The model under review builds one solid part; all positions refer to its coordinate system, in mm. Face numbers are marked on the shaded views. A direction names the side the tool comes from. Round coordinates to 2 decimals unless told otherwise and drop trailing zeros. Write each loop counter-clockwise with the first axis right and the second up, starting at its lowest first coordinate (ties: lowest second). Pieces come first, ordered by that corner, then holes.
Item 1: Clearance check with flat-ended pins moving along their axes: pin 1 Ø0.8 at (x, z) = (-22, -4) entering from -Y; pin 2 Ø2 at (x, y) = (-23, -11) entering from -Z; pin 3 Ø3 at (x, y) = (22.5, -14.5) entering from +Z. State where each tip first meets the part, or that it passes through.
Item 2: Draft analysis for pull direction X (two halves, no side actions). For the marked faces 1, 2 and 3, state which applies: +X half, -X half, draft (parallel to the pull), parting line (faces both ways), or undercut.
Item 3: Add section D-D (x = 31). Give the boundary of the cut face in (y, z).
Item 4: Add section A-A (y = -11.25). Give the boundary of the cut face in (x, z).
Item 5: Add section C-C (y = -21). Give the boundary of the cut face in (x, z), plus the area to 3 significant figures.
Item 6: To check wall thickness, follow L1, parallel to Z at x = -63, y = -11; L2, parallel to X at y = -34, z = 5; L3, parallel to X at y = -39.5, z = 9. State the ranges of each line that lie inside material, in increasing order.
Item 7: Add section B-B (y = -43). Give the boundary of the cut face in (x, z).
Item 8: Machinability: for the marked faces 4 and 5, which of the approach directions +Z, -Z, +X, -X, +Y, -Y give a long, thin tool a straight path to every point of the face, cutting with its end or side? Answer none if there is none.
```python
from build123d import *
from build123d import SkipClean  # not in build123d's __all__

# Parameters (mm, degrees)
F0_W      = 130
F0_H      = 30
F1_DEPTH  = 4
F2_W      = 3.3338604867
F2_H      = 30
F3_DEPTH  = 50
F4_R      = 5.08
F5_R      = 2.5
F6_DEPTH  = 137.16
F7_R      = 4
F7_R_2    = 2.5
F8_DEPTH  = 5
F9_W      = 15
F9_H      = 15
F9_R      = 2.5
F10_DEPTH = 1
F11_W     = 4
F11_H     = 10
F12_DEPTH = 26.0096
F14_DEPTH = 14.224
F16_DEPTH = 6.096
F17_R     = 1.9939
F18_DEPTH = 25.4


# Not quite as in the source:
# - after a boolean that leaves OpenCascade's solid faulty, fix() repairs it
# - a feature names something its author has since deleted; it is built from what else it names


with BuildPart() as f1:
    # F0 (on Front) → F1 (new body)
    with BuildSketch(Plane.XZ):
        Rectangle(F0_W, F0_H)
    extrude(amount=F1_DEPTH)

    # F2 (on face) → F3 (join)
    with BuildSketch(Plane.XZ.offset(4)):
        with Locations((-63.3330697566, 0)):
            Rectangle(F2_W, F2_H)
        with Locations((63.3330697566, 0)):
            Rectangle(F2_W, F2_H)
    extrude(amount=F3_DEPTH)

    # F4
    f4_edges = [f1.edges().sort_by_distance(p)[0] for p in [
        (63.33307, -54, 15),
        (63.33307, -54, -15),
        (-63.33307, -54, -15),
        (-63.33307, -54, 15),
    ]]
    fillet(f4_edges, radius=F4_R)

    # F5 (on face) → F6 (cut)
    with BuildSketch(Plane(origin=(-65, 0, 0), x_dir=(0, -1, 0), z_dir=(-1, 0, 0))):
        with Locations((30, 0)):
            Circle(F5_R)
    extrude(amount=-F6_DEPTH, mode=Mode.SUBTRACT)

    # F7 (on face) → F8 (join)
    with BuildSketch(Plane.YZ.offset(-61.6661395133)):
        with Locations((-30, 0)):
            Circle(F7_R)
        with Locations((-30, 0)):
            Circle(F7_R_2, mode=Mode.SUBTRACT)
    with SkipClean():  # cleaning this boolean's faces spoils the solid; the shape is the same uncleaned
        extrude(amount=F8_DEPTH)

    # F9 (on face) → F10 (cut)
    with BuildSketch(Plane(origin=(61.6661395133, 0, 0), x_dir=(0, -1, 0), z_dir=(-1, 0, 0))):
        with Locations((30, 0)):
            Rectangle(F9_W, F9_H)
        with Locations((30, 0)):
            Circle(F9_R, mode=Mode.SUBTRACT)
    extrude(amount=-F10_DEPTH, mode=Mode.SUBTRACT)

    add(f1.part.fix(), mode=Mode.REPLACE)

    # F11 (on face) → F12 (join)
    with BuildSketch(Plane.XZ.offset(4)):
        with Locations((-22.1996698529, 0)):
            Rectangle(F11_W, F11_H)
        with Locations((22.1996698529, 0)):
            Rectangle(F11_W, F11_H)
    extrude(amount=F12_DEPTH)

    # F13 (on face) → F14 (cut)
    with BuildSketch(Plane.YZ.offset(-20.1996698529)):
        with BuildLine():
            ThreePointArc((-30.0096, -2.4999815679), (-28.2356304242, -1.7711578134), (-27.5, 0))
            ThreePointArc((-27.5, 0), (-28.2356304242, 1.7711578134), (-30.0096, 2.4999815679))
            Line((-30.0096, 2.4999815679), (-30.0096, -2.4999815679))
        make_face()
    extrude(amount=-F14_DEPTH, mode=Mode.SUBTRACT)

    # F15 (on face) → F16 (cut)
    with BuildSketch(Plane.YZ.offset(24.1996698529)):
        with BuildLine():
            Line((-30.0096, 2.4999815679), (-30.0096, -2.4999815679))
            ThreePointArc((-30.0096, -2.4999815679), (-27.5, 0), (-30.0096, 2.4999815679))
        make_face()
    extrude(amount=-F16_DEPTH, mode=Mode.SUBTRACT)

    # F17 (on face) → F18 (cut)
    with BuildSketch(Plane(origin=(-65, 0, 0), x_dir=(0, -1, 0), z_dir=(-1, 0, 0))):
        with Locations((11.25, 0)):
            Circle(F17_R)
    extrude(amount=-F18_DEPTH, mode=Mode.SUBTRACT)


solid = f1.part
```
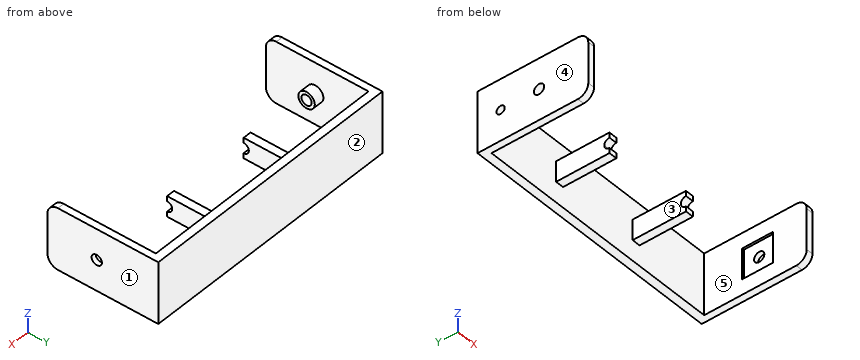
Numbers:
1. pin 1: stops at y = -30.01
1. pin 2: stops at z = -5
1. pin 3: stops at z = 5
2. face 1: +X half
2. face 2: draft
2. face 3: undercut
3. outline: (-4, -15) - (0, -15) - (0, 15) - (-4, 15) - close
4. outline: (-65, -15) - (-61.67, -15) - (-61.67, -1.99) - (-65, -1.99) - close; (-65, 1.99) - (-61.67, 1.99) - (-61.67, 15) - (-65, 15) - close; (-24.2, -5) - (-20.2, -5) - (-20.2, 5) - (-24.2, 5) - close; (20.2, -5) - (24.2, -5) - (24.2, 5) - (20.2, 5) - close; (61.67, -15) - (65, -15) - (65, 15) - (61.67, 15) - close
5. outline: (-65, -15) - (-61.67, -15) - (-61.67, 15) - (-65, 15) - close; (-24.2, -5) - (-20.2, -5) - (-20.2, 5) - (-24.2, 5) - close; (20.2, -5) - (24.2, -5) - (24.2, 5) - (20.2, 5) - close; (61.67, -15) - (65, -15) - (65, 15) - (61.67, 15) - close
5. area: 280 mm2
6. L1: z = -15 to -1.98, 1.98 to 15
6. L2: x = -65 to -61.67, 62.67 to 65
6. L3: x = -65 to -61.67, 61.67 to 65
7. outline: (-65, -15) - (-61.67, -15) - (-61.67, 15) - (-65, 15) - close; (61.67, -15) - (65, -15) - (65, 15) - (61.67, 15) - close
8. face 4: +Z, -Z, -X, +Y, -Y
8. face 5: +Z, -Z, -Y
